Geometry: see drawing. Coordinates: mm, zero at the bounding-box minimum. A direction names the side the tool comes from. Coordinates: 2 decimals unless noted, no trailing zeros. Write each loop counter-clockwise with the first axis right and the second up, starting at its lowest first coordinate (ties: lowest second). Pieces come first, ordered by that corner, then holes. Notation, with made-up numbers: M -34.75,36.5 L -11.75,36.5 A30 ccw -11.75,60.5 Z; hole C -28.5,47.25 d1. An arc over 180 degrees is marked long. Answer as CSV lines item,"result". Start each with the question number.
1. Reachability of the marked faces 1, 2 and 3 from +Z, -Z, +X, -X, +Y, -Y: full face, straight path, thin tool, end or side. Return the list, or none.
2. Contact query for flat-ended pins moving along their axis: pin 1 Ø8 at (x, z) = (29, 42) entering from -Y; pin 2 Ø8 at (x, y) = (16, 69) entering from +Z; pin 3 Ø13 at (y, z) = (43, 16.5) entering from -X; pin 4 Ø16 at (y, z) = (43, 43) entering from +X. Output: stop coordinate, or through.
3. Section C-C on x = 25. Return the cut outline in (y, z), plus the area to 3 significant figures.
4. Line query: probe 1 along Y at (x, z) = (20, 43); probe 2 along Y at (x, z) = (31.5, 38); probe 3 along X at (y, z) = (31, 72). Output: solid intervals per line, ascending. Write a range as [from, to].
5. Section A-A on z = 43. Count the separate pieces of the cut face and the enclosed holes in it, plus the area to 3 significant figures.
6. Section D-D on x = 6. Return the cut outline in (y, z).
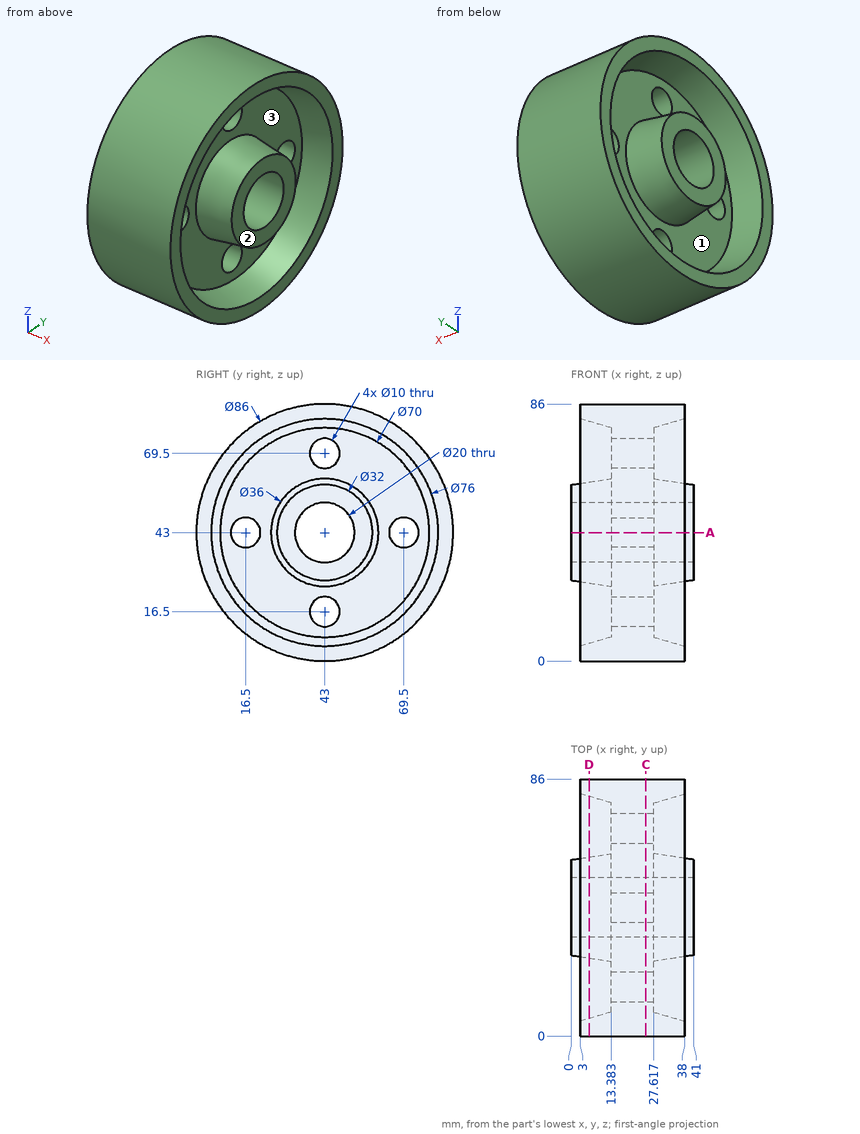
Values:
1,face 1,"-X"
1,face 2,"+Z, -Z, +X, +Y, -Y"
1,face 3,"+X"
2,pin 1,"y = 0"
2,pin 2,"z = 79.95"
2,pin 3,"x = 13.38"
2,pin 4,"through"
3,outline,"C 43,43 d86; hole C 16.5,43 d10; hole C 43,43 d20; hole C 43,16.5 d10; hole C 43,69.5 d10; hole C 69.5,43 d10"
3,area,"5,180 mm²"
4,probe 1,"[0, 11.5], [21.5, 33], [53, 64.5], [74.5, 86]"
4,probe 2,"[0.29, 7.23], [26.31, 34.34], [51.66, 59.69], [78.77, 85.71]"
4,probe 3,"[13.38, 27.62]"
5,separate pieces,"4"
5,enclosed holes,"0"
5,area,"1,300 mm²"
6,outline,"C 43,43 d86; C 43,43 d33.79; hole C 43,43 d74.27; hole C 43,43 d20"
